```python
from build123d import *

# Parameters (mm, degrees)
RESSALTO_EXTRUS_O1_DEPTH   = 15
ESBO_O1_3_R                = 1.5
RESSALTO_EXTRUS_O2_DEPTH   = 12
ESBO_O1_4_R                = 1.35
RESSALTO_EXTRUS_O3_DEPTH   = 12
CORTE_EXTRUS_O1_DEPTH      = 38.624816903
CORTE_EXTRUS_O1_DEPTH_BACK = 38.624816903


with BuildPart() as part:
    # Esboço1 → Ressalto-extrusão1 (new body)
    with BuildSketch(Plane.XY):
        with BuildLine():
            ThreePointArc((0, -3.4), (-3.4, 0), (0, 3.4))
            Line((0, 3.4), (4.942053961, 3.4))
            ThreePointArc((4.942053961, 3.4), (5.218299225, 4.96081936), (5.596969896, 6.5))
            Line((5.596969896, 6.5), (0, 6.5))
            ThreePointArc((0, 6.5), (-0.834966341, 6.446148556), (-1.656097561, 6.285486526))
            ThreePointArc((-1.656097561, 6.285486526), (-6.446148556, -0.834966341), (0, -6.5))
            Line((0, -6.5), (1.464912337, -6.5))
            Line((1.464912337, -6.5), (5.596969896, -6.5))
            ThreePointArc((5.596969896, -6.5), (5.218299225, -4.96081936), (4.942053961, -3.4))
            Line((4.942053961, -3.4), (0, -3.4))
        make_face()
    extrude(amount=RESSALTO_EXTRUS_O1_DEPTH)

    # Esboço1<3> → Ressalto-extrusão2 (add)
    with BuildSketch(Plane.XY):
        with BuildLine():
            Line((4.942053961, 3.4), (0, 3.4))
            ThreePointArc((0, 3.4), (-3.4, 0), (0, -3.4))
            Line((0, -3.4), (4.942053961, -3.4))
            ThreePointArc((4.942053961, -3.4), (4.7, 0), (4.942053961, 3.4))
        make_face()
        Circle(ESBO_O1_3_R, mode=Mode.SUBTRACT)
    extrude(amount=RESSALTO_EXTRUS_O2_DEPTH)

    # Esboço1<4> → Ressalto-extrusão3 (add)
    # profile 1 of 2: a face of its own
    with BuildSketch(Plane.XY):
        with BuildLine():
            Line((0, 6.5), (5.596969896, 6.5))
            ThreePointArc((5.596969896, 6.5), (10.608614203, 15.770280909), (19.108336953, 22))
            Line((19.108336953, 22), (4.96620133, 27))
            Line((4.96620133, 27), (3.299534663, 22.285954792))
            Line((3.299534663, 22.285954792), (6.154368486, 21.276618614))
            ThreePointArc((6.154368486, 21.276618614), (1.207605686, 14.323695574), (-1.656097561, 6.285486526))
            ThreePointArc((-1.656097561, 6.285486526), (-0.834966341, 6.446148556), (0, 6.5))
        make_face()
        with Locations((6.961295121, 23.642977396)):
            Circle(ESBO_O1_4_R, mode=Mode.SUBTRACT)
        with Locations((13.560958412, 21.309644063)):
            Circle(ESBO_O1_4_R, mode=Mode.SUBTRACT)
    # profile 2 of 2: a face of its own
    with BuildSketch(Plane.XY):
        with BuildLine():
            ThreePointArc((7.915390309, -12), (6.584536367, -9.322353153), (5.596969896, -6.5))
            Line((5.596969896, -6.5), (1.464912337, -6.5))
            ThreePointArc((1.464912337, -6.5), (2.686390311, -10.358190524), (4.451288694, -14))
            Line((4.451288694, -14), (7.915390309, -12))
        make_face()
    extrude(amount=RESSALTO_EXTRUS_O3_DEPTH)

    # Esboço2 → Corte-extrusão1 (cut, two sides: drawn at the far end of the back side and taken through both)
    with BuildSketch(Plane(origin=(-4.070880192, 1.439273495, 0), x_dir=(0, 0, 1), z_dir=(-0.9428090415820632, 0.33333333333333404, 0)).offset(-CORTE_EXTRUS_O1_DEPTH_BACK)):
        Polygon((0, -11.715563684), (9, -11.715563684), (9, 13.111244566), (0, 22.111244566), align=None)
        Polygon((4.242640687, 27.111244566), (4.242640687, 22.111244566), (12, 14.353885253), (12, 27.111244566), align=None)
    extrude(amount=CORTE_EXTRUS_O1_DEPTH + CORTE_EXTRUS_O1_DEPTH_BACK, mode=Mode.SUBTRACT)


solid = part.part
```
Can you work these out from the model? Positions are in its coordinate system, mm. A direction names the side the tool comes from. Coordinates: 2 decimals unless noted, no trailing zeros. Loops run counter-clockwise (first coordinate to the right, second up) from the corner with the lowest first, then second, coordinate; pieces in that order, holes last.
1) For pin 1 (7 mm diameter, centred on x = -1.5, y = -3.5, fed in from -Z); pin 2 (0.9 mm diameter, centred on x = 2, z = 14, fed in from +Y); pin 3 (1.9 mm diameter, centred on x = 3, y = -8.5, fed in from +Z), each with a flat end and sliding along its axis, tell me the tip position at first contact or that it passes through.
2) Imagine slicing it at B-B on z = 3. List the corners of the cut face in (x, y) for me, plus the area to 3 significant figures.
3) Imagine slicing it at C-C on x = 11. List the corners of the cut face in (y, z) for me.
4) Imagine slicing it at A-A on y = 0. List the corners of the cut face in (x, z) for me.
5) I need wall thicknesses on probe 1 along Y at (x, z) = (1.75, 13.5); probe 2 along Z at (x, y) = (-1, -4.5); probe 3 along Z at (x, y) = (3.5, 7). Which ranges of each line are inside material? Lowest first, please.
6) Which directions (+Z, -Z, +X, -X, +Y, -Y) give clear straight access to the entire face, cutting with the end or side of a thin tool? Please do faces 1 (the flat face through (10, 23, 4.243)), 2 (the flat face through (3, -3.4, 13)), 3 (the flat face through (5, -10, 12)).
7) Thinking about a two-plate mould opening in X: for faces 4 (the flat face through (4.707, 21.788, 2.092)), 5 (the flat face through (2, 3, 9)), 6 (the cylindrical face through (6.786, 24.981, 2.092)), which applies, pulls with the +X half, pulls with the -X half, needs draft (parallel to the pull), parting line crosses it, or undercut?
8) Imagine slicing it at D-D on z = 5. List the corners of the cut face in (x, y) for me.
Completed:
1. pin 1: stops at z = 9
1. pin 2: stops at y = 6.5
1. pin 3: stops at z = 12
2. outline: (3.3, 22.29) - (6.15, 21.28) arc R31 ccw to (4.07, 18.83) - (11.12, 16.34) arc R24 cw to (19.11, 22) - (4.97, 27) - close; hole circle Ø2.7 at (6.96, 23.64); hole circle Ø2.7 at (13.56, 21.31)
2. area: 75.4 mm2
3. outline: (16.21, 3.16) - (19.56, 0) - (24.87, 0) - (24.87, 4.24) - (19.56, 4.24) - (16.21, 7.41) - close
4. outline: (-6.5, 9) - (-1.5, 9) - (-1.5, 12) - (-3.4, 12) - (-3.4, 15) - (-6.5, 15) - close; (1.5, 9) - (4.7, 9) - (4.7, 12) - (1.5, 12) - close
5. probe 1: y = -6.5 to -3.4, 3.4 to 6.5
5. probe 2: z = 9 to 15
5. probe 3: z = 9 to 12
6. face 1: +Z, +X, +Y
6. face 2: +Z, +X
6. face 3: +Z, +X, -X, -Y
7. face 4: pulls with the -X half
7. face 5: needs draft
7. face 6: undercut
8. outline: (2.87, 17.14) - (9.73, 14.71) arc R24 cw to (12.92, 18.08) - (5.6, 20.67) arc R31 ccw to start
